from build123d import *

# Parameters (mm, degrees)
SKETCH1_R           = 34.470588235
BOSS_EXTRUDE1_DEPTH = 2
SKETCH2_W           = 4
SKETCH2_H           = 10
CUT_EXTRUDE1_DEPTH  = 49.912604782


with BuildPart() as part:
    # Sketch1 → Boss-Extrude1 (new, symmetric)
    with BuildSketch(Plane(origin=(0, 0, 0), x_dir=(0, 0, -1), z_dir=(1, 0, 0))):
        Circle(SKETCH1_R)
    extrude(amount=BOSS_EXTRUDE1_DEPTH, both=True)

    # Sketch2 → Cut-Extrude1 (cut, through all)
    with BuildSketch(Plane(origin=(2, 0, 0), x_dir=(0, 0, -1), z_dir=(1, 0, 0))):
        with Locations((6, 24.529411765)):
            Rectangle(SKETCH2_W, SKETCH2_H)
        with Locations((6, -0.470588235)):
            Rectangle(SKETCH2_W, SKETCH2_H)
        with Locations((6, -25.470588235)):
            Rectangle(SKETCH2_W, SKETCH2_H)
    cut_extrude1 = extrude(amount=-CUT_EXTRUDE1_DEPTH, mode=Mode.SUBTRACT)

    # Mirror1: Cut-Extrude1 across plane
    add(cut_extrude1.mirror(Plane.XY), mode=Mode.SUBTRACT)


solid = part.part
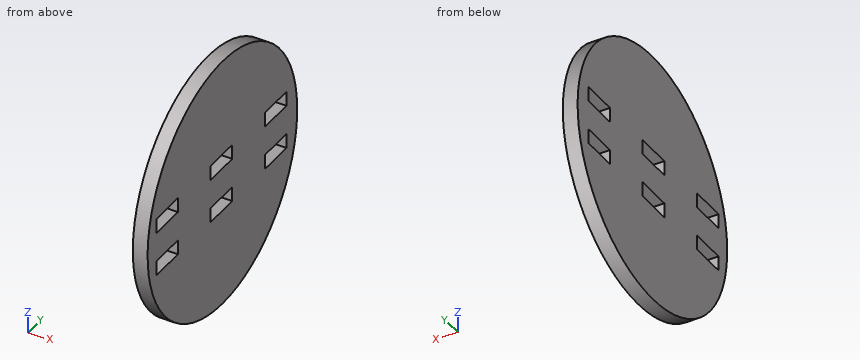
Source: CAD feature listing. Evaluate the final solid. Frame: model axes, mm. Round coordinates to 2 decimals unless told otherwise and drop trailing zeros. Order: outer loops, then holes, each group sorted by start corner. A loop starts at its lowest first (then second) coordinate and runs counter-clockwise, first axis right, second up. Notation, with made-up numbers: (12.5, 49.5) - (59.5, 49.5) arc R15 ccw to (59.5, 78.5) - close; hole circle Ø9 at (56.25, 3.5). An arc over 180 degrees is marked (long way). Use a Markdown table: item, result. Add a question column.
1. Section query C-C (z = 7). Return the cut outline in (x, y), then the cut area to 3 significant figures.
2. First-contact query: pin 1 (1.2 mm diameter, centred on x = -0.5, z = 5, fed in from +Y); pin 2 (2 mm diameter, centred on x = -1, y = -2.5, fed in from -Z); pin 3 (1.5 mm diameter, centred on x = 1, z = 8.5, fed in from +Y). Flat tips, straight axial feed; report the tip coordinate or a pass-through.
3. Section query B-B (x = 1.4). Return the cut outline in (y, z), then the cut area to 3 significant figures.
4. Line query: probe 1 along Z at (x, y) = (-1.6, 25); probe 2 along Z at (x, y) = (0.25, -27.5); probe 3 along Y at (x, z) = (1.2, 5). Output: solid intervals per line, ascending.
5. Section query A-A (y = 0). Return the cut outline in (x, z).
6. Section query D-D (z = -12). Return the cut outline in (x, y), then the cut area to 3 significant figures.
Derived:
| question | item | result |
|---|---|---|
| 1 | outline | (-2, -33.75) - (2, -33.75) - (2, -30.47) - (-2, -30.47) - close; (-2, -20.47) - (2, -20.47) - (2, -5.47) - (-2, -5.47) - close; (-2, 4.53) - (2, 4.53) - (2, 19.53) - (-2, 19.53) - close; (-2, 29.53) - (2, 29.53) - (2, 33.75) - (-2, 33.75) - close |
| 1 | area | 150 mm2 |
| 2 | pin 1 | y = 34.19 |
| 2 | pin 2 | z = -34.44 |
| 2 | pin 3 | y = 33.59 |
| 3 | outline | circle Ø68.94 at (0, 0); hole (-30.47, -8) - (-20.47, -8) - (-20.47, -4) - (-30.47, -4) - close; hole (-30.47, 4) - (-20.47, 4) - (-20.47, 8) - (-30.47, 8) - close; hole (-5.47, -8) - (4.53, -8) - (4.53, -4) - (-5.47, -4) - close; hole (-5.47, 4) - (4.53, 4) - (4.53, 8) - (-5.47, 8) - close; hole (19.53, -8) - (29.53, -8) - (29.53, -4) - (19.53, -4) - close; hole (19.53, 4) - (29.53, 4) - (29.53, 8) - (19.53, 8) - close |
| 3 | area | 3,490 mm2 |
| 4 | probe 1 | -23.73 to -8, -4 to 4, 8 to 23.73 |
| 4 | probe 2 | -20.78 to -8, -4 to 4, 8 to 20.78 |
| 4 | probe 3 | -34.11 to -30.47, -20.47 to -5.47, 4.53 to 19.53, 29.53 to 34.11 |
| 5 | outline | (-2, -34.47) - (2, -34.47) - (2, -8) - (-2, -8) - close; (-2, -4) - (2, -4) - (2, 4) - (-2, 4) - close; (-2, 8) - (2, 8) - (2, 34.47) - (-2, 34.47) - close |
| 6 | outline | (-2, -32.31) - (2, -32.31) - (2, 32.31) - (-2, 32.31) - close |
| 6 | area | 259 mm2 |
